Check sheet for the modelled part. Datum: model origin and axes. Units: mm. Round coordinates to 2 decimals unless told otherwise and drop trailing zeros. Loops run counter-clockwise (first coordinate to the right, second up) from the corner with the lowest first, then second, coordinate; pieces in that order, holes last. Notation, with made-up numbers: (56, 51) -> (92, 51) arc R30 cw to (92, 78) -> close; hole circle Ø7 at (41, 40). An arc over 180 degrees is marked (long way). One line per item, written item: value. Start each with the question number.
1. Cross-section at C-C on x = 6.5. Record the cut outline in (y, z).
2. Cross-section at A-A on x = -72.5. Record the cut outline in (y, z), then the cut area to 3 significant figures.
3. Material ranges on L1, parallel to Y at x = 229, z = 3.4; L2, parallel to Z at x = 128, y = 24.5; L3, parallel to Y at x = 17, z = 2.6, recorded low to high.
4. Cross-section at B-B on y = 22. Record the cut outline in (x, z).
5. Go/stop test with a flat-tipped pin: pin 1 (5.5 mm diameter, centred on x = 183, y = 21.5, fed in from +Z). Record where the tip stops, or that it passes through.
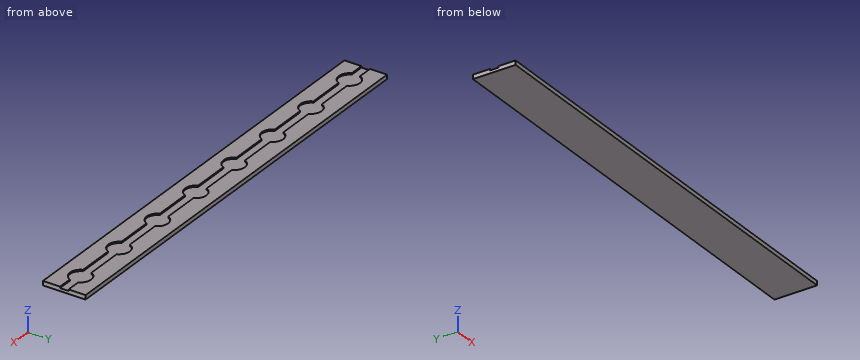
from build123d import *

# Parameters (mm, degrees)
F0_W     = 398.78
F0_H     = 38.1
F1_DEPTH = 3.81
F2_R     = 9.525
F3_DEPTH = 1.27
F5_DEPTH = 1.27


with BuildPart() as f1:
    # F0 (on Top) → F1 (new body)
    with BuildSketch(Plane.XY):
        with Locations((85.0978558012, 21.4591654949)):
            Rectangle(F0_W, F0_H)
    extrude(amount=F1_DEPTH)

    # F2 (on face) → F3 (cut)
    with BuildSketch(Plane.XY.offset(3.81)):
        with Locations((-92.7021441988, 21.4591654949)):
            Circle(F2_R)
        with Locations((-41.9021441988, 21.4591654949)):
            Circle(F2_R)
        with Locations((8.8978558012, 21.4591654949)):
            Circle(F2_R)
        with Locations((59.6978558012, 21.4591654949)):
            Circle(F2_R)
        with Locations((110.4978558012, 21.4591654949)):
            Circle(F2_R)
        with Locations((161.2978558012, 21.4591654949)):
            Circle(F2_R)
        with Locations((212.0978558012, 21.4591654949)):
            Circle(F2_R)
        with Locations((262.8978558012, 21.4591654949)):
            Circle(F2_R)
    extrude(amount=-F3_DEPTH, mode=Mode.SUBTRACT)

    # F4 (on face) → F5 (cut)
    with BuildSketch(Plane.XY.offset(3.81)):
        with BuildLine():
            Line((-101.4319508977, 25.2691654949), (-114.2921441988, 25.2691654949))
            Line((-114.2921441988, 25.2691654949), (-114.2921441988, 17.6491654949))
            Line((-114.2921441988, 17.6491654949), (-101.4319508977, 17.6491654949))
            ThreePointArc((-101.4319508977, 17.6491654949), (-102.2271441988, 21.4591654949), (-101.4319508977, 25.2691654949))
        make_face()
        with BuildLine():
            Line((-83.9723374999, 25.2691654949), (-101.4319508977, 25.2691654949))
            ThreePointArc((-101.4319508977, 25.2691654949), (-102.2271441988, 21.4591654949), (-101.4319508977, 17.6491654949))
            Line((-101.4319508977, 17.6491654949), (-83.9723374999, 17.6491654949))
            ThreePointArc((-83.9723374999, 17.6491654949), (-83.3780615681, 19.5131161387), (-83.1771441988, 21.4591654949))
            ThreePointArc((-83.1771441988, 21.4591654949), (-83.3780615681, 23.405214851), (-83.9723374999, 25.2691654949))
        make_face()
        with BuildLine():
            Line((-50.6319508977, 25.2691654949), (-83.9723374999, 25.2691654949))
            ThreePointArc((-83.9723374999, 25.2691654949), (-83.3780615681, 23.405214851), (-83.1771441988, 21.4591654949))
            ThreePointArc((-83.1771441988, 21.4591654949), (-83.3780615681, 19.5131161387), (-83.9723374999, 17.6491654949))
            Line((-83.9723374999, 17.6491654949), (-50.6319508977, 17.6491654949))
            ThreePointArc((-50.6319508977, 17.6491654949), (-51.4271441988, 21.4591654949), (-50.6319508977, 25.2691654949))
        make_face()
        with BuildLine():
            Line((-33.1723374999, 25.2691654949), (-50.6319508977, 25.2691654949))
            ThreePointArc((-50.6319508977, 25.2691654949), (-51.4271441988, 21.4591654949), (-50.6319508977, 17.6491654949))
            Line((-50.6319508977, 17.6491654949), (-33.1723374999, 17.6491654949))
            ThreePointArc((-33.1723374999, 17.6491654949), (-32.5780615681, 19.5131161387), (-32.3771441988, 21.4591654949))
            ThreePointArc((-32.3771441988, 21.4591654949), (-32.5780615681, 23.405214851), (-33.1723374999, 25.2691654949))
        make_face()
        with BuildLine():
            Line((284.4878558012, 17.6491654949), (284.4878558012, 25.2691654949))
            Line((284.4878558012, 25.2691654949), (271.6276625001, 25.2691654949))
            ThreePointArc((271.6276625001, 25.2691654949), (272.2219384319, 23.405214851), (272.4228558012, 21.4591654949))
            ThreePointArc((272.4228558012, 21.4591654949), (272.2219384319, 19.5131161387), (271.6276625001, 17.6491654949))
            Line((271.6276625001, 17.6491654949), (284.4878558012, 17.6491654949))
        make_face()
        with BuildLine():
            Line((0.1680491023, 25.2691654949), (-33.1723374999, 25.2691654949))
            ThreePointArc((-33.1723374999, 25.2691654949), (-32.5780615681, 23.405214851), (-32.3771441988, 21.4591654949))
            ThreePointArc((-32.3771441988, 21.4591654949), (-32.5780615681, 19.5131161387), (-33.1723374999, 17.6491654949))
            Line((-33.1723374999, 17.6491654949), (0.1680491023, 17.6491654949))
            ThreePointArc((0.1680491023, 17.6491654949), (-0.6271441988, 21.4591654949), (0.1680491023, 25.2691654949))
        make_face()
        with BuildLine():
            Line((17.6276625001, 25.2691654949), (0.1680491023, 25.2691654949))
            ThreePointArc((0.1680491023, 25.2691654949), (-0.6271441988, 21.4591654949), (0.1680491023, 17.6491654949))
            Line((0.1680491023, 17.6491654949), (17.6276625001, 17.6491654949))
            ThreePointArc((17.6276625001, 17.6491654949), (18.2219384319, 19.5131161387), (18.4228558012, 21.4591654949))
            ThreePointArc((18.4228558012, 21.4591654949), (18.2219384319, 23.405214851), (17.6276625001, 25.2691654949))
        make_face()
        with BuildLine():
            ThreePointArc((254.1680491023, 17.6491654949), (253.3728558012, 21.4591654949), (254.1680491023, 25.2691654949))
            Line((254.1680491023, 25.2691654949), (220.8276625001, 25.2691654949))
            ThreePointArc((220.8276625001, 25.2691654949), (221.4219384319, 23.405214851), (221.6228558012, 21.4591654949))
            ThreePointArc((221.6228558012, 21.4591654949), (221.4219384319, 19.5131161387), (220.8276625001, 17.6491654949))
            Line((220.8276625001, 17.6491654949), (254.1680491023, 17.6491654949))
        make_face()
        with BuildLine():
            Line((50.9680491023, 25.2691654949), (17.6276625001, 25.2691654949))
            ThreePointArc((17.6276625001, 25.2691654949), (18.2219384319, 23.405214851), (18.4228558012, 21.4591654949))
            ThreePointArc((18.4228558012, 21.4591654949), (18.2219384319, 19.5131161387), (17.6276625001, 17.6491654949))
            Line((17.6276625001, 17.6491654949), (50.9680491023, 17.6491654949))
            ThreePointArc((50.9680491023, 17.6491654949), (50.1728558012, 21.4591654949), (50.9680491023, 25.2691654949))
        make_face()
        with BuildLine():
            ThreePointArc((221.6228558012, 21.4591654949), (221.4219384319, 23.405214851), (220.8276625001, 25.2691654949))
            Line((220.8276625001, 25.2691654949), (203.3680491023, 25.2691654949))
            ThreePointArc((203.3680491023, 25.2691654949), (202.5728558012, 21.4591654949), (203.3680491023, 17.6491654949))
            Line((203.3680491023, 17.6491654949), (220.8276625001, 17.6491654949))
            ThreePointArc((220.8276625001, 17.6491654949), (221.4219384319, 19.5131161387), (221.6228558012, 21.4591654949))
        make_face()
        with BuildLine():
            Line((68.4276625001, 25.2691654949), (50.9680491023, 25.2691654949))
            ThreePointArc((50.9680491023, 25.2691654949), (50.1728558012, 21.4591654949), (50.9680491023, 17.6491654949))
            Line((50.9680491023, 17.6491654949), (68.4276625001, 17.6491654949))
            ThreePointArc((68.4276625001, 17.6491654949), (69.0219384319, 19.5131161387), (69.2228558012, 21.4591654949))
            ThreePointArc((69.2228558012, 21.4591654949), (69.0219384319, 23.405214851), (68.4276625001, 25.2691654949))
        make_face()
        with BuildLine():
            ThreePointArc((203.3680491023, 17.6491654949), (202.5728558012, 21.4591654949), (203.3680491023, 25.2691654949))
            Line((203.3680491023, 25.2691654949), (170.0276625001, 25.2691654949))
            ThreePointArc((170.0276625001, 25.2691654949), (170.6219384319, 23.405214851), (170.8228558012, 21.4591654949))
            ThreePointArc((170.8228558012, 21.4591654949), (170.6219384319, 19.5131161387), (170.0276625001, 17.6491654949))
            Line((170.0276625001, 17.6491654949), (203.3680491023, 17.6491654949))
        make_face()
        with BuildLine():
            Line((101.7680491023, 25.2691654949), (68.4276625001, 25.2691654949))
            ThreePointArc((68.4276625001, 25.2691654949), (69.0219384319, 23.405214851), (69.2228558012, 21.4591654949))
            ThreePointArc((69.2228558012, 21.4591654949), (69.0219384319, 19.5131161387), (68.4276625001, 17.6491654949))
            Line((68.4276625001, 17.6491654949), (101.7680491023, 17.6491654949))
            ThreePointArc((101.7680491023, 17.6491654949), (100.9728558012, 21.4591654949), (101.7680491023, 25.2691654949))
        make_face()
        with BuildLine():
            ThreePointArc((170.8228558012, 21.4591654949), (170.6219384319, 23.405214851), (170.0276625001, 25.2691654949))
            Line((170.0276625001, 25.2691654949), (152.5680491023, 25.2691654949))
            ThreePointArc((152.5680491023, 25.2691654949), (151.7728558012, 21.4591654949), (152.5680491023, 17.6491654949))
            Line((152.5680491023, 17.6491654949), (170.0276625001, 17.6491654949))
            ThreePointArc((170.0276625001, 17.6491654949), (170.6219384319, 19.5131161387), (170.8228558012, 21.4591654949))
        make_face()
        with BuildLine():
            Line((119.2276625001, 25.2691654949), (101.7680491023, 25.2691654949))
            ThreePointArc((101.7680491023, 25.2691654949), (100.9728558012, 21.4591654949), (101.7680491023, 17.6491654949))
            Line((101.7680491023, 17.6491654949), (119.2276625001, 17.6491654949))
            ThreePointArc((119.2276625001, 17.6491654949), (119.8219384319, 19.5131161387), (120.0228558012, 21.4591654949))
            ThreePointArc((120.0228558012, 21.4591654949), (119.8219384319, 23.405214851), (119.2276625001, 25.2691654949))
        make_face()
        with BuildLine():
            ThreePointArc((152.5680491023, 17.6491654949), (151.7728558012, 21.4591654949), (152.5680491023, 25.2691654949))
            Line((152.5680491023, 25.2691654949), (119.2276625001, 25.2691654949))
            ThreePointArc((119.2276625001, 25.2691654949), (119.8219384319, 23.405214851), (120.0228558012, 21.4591654949))
            ThreePointArc((120.0228558012, 21.4591654949), (119.8219384319, 19.5131161387), (119.2276625001, 17.6491654949))
            Line((119.2276625001, 17.6491654949), (152.5680491023, 17.6491654949))
        make_face()
    extrude(amount=-F5_DEPTH, mode=Mode.SUBTRACT)


solid = f1.part
Taken from the geometry:
1. outline: (2.41, 0) -> (40.51, 0) -> (40.51, 3.81) -> (30.68, 3.81) -> (30.68, 2.54) -> (12.24, 2.54) -> (12.24, 3.81) -> (2.41, 3.81) -> close
2. outline: (2.41, 0) -> (40.51, 0) -> (40.51, 3.81) -> (25.27, 3.81) -> (25.27, 2.54) -> (17.65, 2.54) -> (17.65, 3.81) -> (2.41, 3.81) -> close
2. area: 135 mm2
3. L1: y = 2.41 to 17.65, 25.27 to 40.51
3. L2: z = 0 to 2.54
3. L3: y = 2.41 to 16.45, 26.47 to 40.51
4. outline: (-114.29, 0) -> (284.49, 0) -> (284.49, 2.54) -> (-114.29, 2.54) -> close
5. pin 1: stops at z = 2.54
